Source: CAD feature listing. Evaluate the final solid. Frame: model axes, mm. Face numbers are marked on the shaded views. A direction names the side the tool comes from. Coordinates: 2 decimals unless noted, no trailing zeros. Order: outer loops, then holes, each group sorted by start corner. A loop starts at its lowest first (then second) coordinate and runs counter-clockwise, first axis right, second up.
Item 1: Section B-B on x = 4.75. Return the cut outline in (y, z), then the cut area to 3 significant figures.
Item 2: Section C-C on z = -6.25. Return the cut outline in (x, y), then the cut area to 3 significant figures.
Item 3: Mould query, pull axis X, two halves, no side actions, for the marked faces 1, 2, 3 and 4. Classes: released by +X, released by -X, zero draft, split by the parting line, or undercut.
Item 4: Ray query, line 1 (X direction, y = 8, z = -3.25); line 2 (Y direction, x = 4.75, z = -1.15); line 3 (X direction, y = -7.75, z = -2). Return the intervals inside material, ascending.
Item 5: Reachability of the marked faces 5 and 6 from +Z, -Z, +X, -X, +Y, -Y: full face, straight path, thin tool, end or side. Return the list, or none.
Item 6: Section D-D on x = -9.5. Return the cut outline in (y, z).
Item 7: Contact query for flat-ended pins moving along their axis: P1, Ø4, axis at y = -0.5, z = -5, coming from the +X side; P2, Ø5.5, axis at x = 0, y = 0, coming from the -Z side (3 decimals); P3, Ø4, axis at x = 9.5, y = 0, coming from the -Z side; P4, Ø5, axis at y = -7.5, z = -1.5, coming from the +X side. Output: stop coordinate, or through.
Item 8: Section A-A on y = 0. Return the cut outline in (x, z).
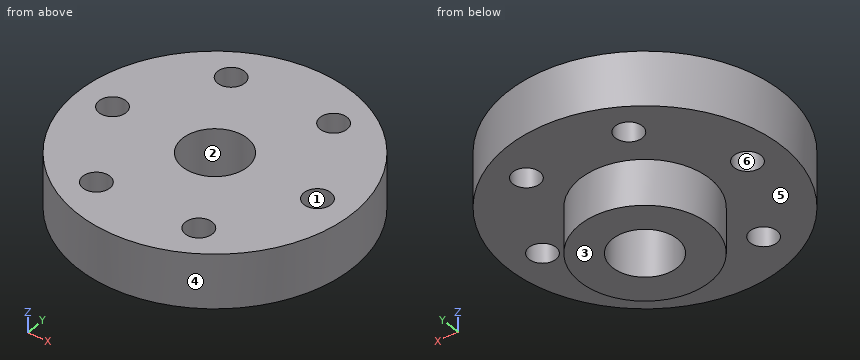
from build123d import *

# Parameters (mm, degrees)
TAP_DRILL_FOR_M3X0_5_TAP1_D     = 2.5
TAP_DRILL_FOR_M3X0_5_TAP1_DEPTH = 10
TAP_DRILL_FOR_M3X0_5_TAP1_TIP   = 0.751075774


with BuildPart() as part:
    # Sketch1 → Revolve1 (revolve)
    with BuildSketch(Plane(origin=(0, 0, 0), x_dir=(0, 0, -1), z_dir=(1, 0, 0))):
        Polygon((0, 3), (0, 12.7), (5, 12.7), (5, 6), (9.2, 6), (9.2, 3), align=None)
    revolve(axis=Axis((0, 0, 50.268991478), (0, 0, -1)))

    # Tap Drill for M3x0.5 Tap1
    with Locations(Plane.XY):
        with Locations((-4.75, 8.227241336), (4.75, 8.227241336), (9.5, 0), (4.75, -8.227241336), (-4.75, -8.227241336), (-9.5, 0)):
            Hole(TAP_DRILL_FOR_M3X0_5_TAP1_D / 2, depth=TAP_DRILL_FOR_M3X0_5_TAP1_DEPTH)
            with Locations((0, 0, -(TAP_DRILL_FOR_M3X0_5_TAP1_DEPTH + TAP_DRILL_FOR_M3X0_5_TAP1_TIP / 2))):  # 118° drill point
                Cone(0, TAP_DRILL_FOR_M3X0_5_TAP1_D / 2, TAP_DRILL_FOR_M3X0_5_TAP1_TIP, mode=Mode.SUBTRACT)


solid = part.part
Answer list:
1. outline: (-11.78, -5) - (-9.48, -5) - (-9.48, 0) - (-11.78, 0) - close; (-6.98, -5) - (-3.67, -5) - (-3.67, -9.2) - (3.67, -9.2) - (3.67, -5) - (6.98, -5) - (6.98, 0) - (-6.98, 0) - close; (9.48, -5) - (11.78, -5) - (11.78, 0) - (9.48, 0) - close
1. area: 124 mm2
2. outline: circle Ø12 at (0, 0); hole circle Ø6 at (0, 0)
2. area: 84.8 mm2
3. face 1: undercut
3. face 2: undercut
3. face 3: zero draft
3. face 4: split by the parting line
4. line 1: x = -9.86 to -5.98, -3.52 to 3.52, 5.98 to 9.86
4. line 2: y = -11.78 to -9.48, -6.98 to 6.98, 9.48 to 11.78
4. line 3: x = -10.06 to -5.91, -3.59 to 3.59, 5.91 to 10.06
5. face 5: -Z
5. face 6: +Z, -Z
6. outline: (-8.43, -5) - (-1.25, -5) - (-1.25, 0) - (-8.43, 0) - close; (1.25, -5) - (8.43, -5) - (8.43, 0) - (1.25, 0) - close
7. P1: stops at x = 12.7
7. P2: passes through
7. P3: stops at z = -5
7. P4: stops at x = 11.67
8. outline: (-12.7, -5) - (-10.75, -5) - (-10.75, 0) - (-12.7, 0) - close; (-8.25, -5) - (-6, -5) - (-6, -9.2) - (-3, -9.2) - (-3, 0) - (-8.25, 0) - close; (3, -9.2) - (6, -9.2) - (6, -5) - (8.25, -5) - (8.25, 0) - (3, 0) - close; (10.75, -5) - (12.7, -5) - (12.7, 0) - (10.75, 0) - close
